Autodesk Inventor part; units mm, degrees
ref_plane "YZ Plane" through (0, 0, 0) normal (1, 0, 0) x (0, 1, 0)
ref_plane "XZ Plane" through (0, 0, 0) normal (0, 1, 0) x (-1, 0, 0)
ref_plane "XY Plane" through (0, 0, 0) normal (0, 0, 1) x (1, 0, 0)
sketch "Sketch1" plane through (0, 0, 0) normal (0, 0, 1) x (1, 0, 0)
  line L0 (-230, 170) -> (230, 170)
  line L1 (230, 170) -> (230, -170)
  line L2 (230, -170) -> (-230, -170)
  line L3 (-230, -170) -> (-230, 170)
  line L4 (130, 170) -> (230, 170)
  line L5 (230, 170) -> (230, -170)
  line L6 (230, -170) -> (130, -170)
  line L7 (130, -170) -> (130, 170)
  line L8 (-230, 170) -> (-130, 170)
  line L9 (-130, 170) -> (-130, -170)
  line L10 (-130, -170) -> (-230, -170)
  line L11 (-230, -170) -> (-230, 170)
  line L12 (-230, 170) -> (230, 170)
  line L13 (230, 170) -> (230, 95)
  line L14 (230, 95) -> (-230, 95)
  line L15 (-230, 95) -> (-230, 170)
  line L16 (-230, -95) -> (230, -95)
  line L17 (230, -95) -> (230, -170)
  line L18 (230, -170) -> (-230, -170)
  line L19 (-230, -170) -> (-230, -95)
  point P0 (0, 0)
  dimension "d0" = 460
  dimension "d1" = 340
  dimension "d2" = 170
  dimension "d3" = 230
  dimension "d4" = 100
  dimension "d5" = 100
  dimension "d6" = 75
  dimension "d7" = 75
extrude "Extrusion1" add sketch "Sketch1" along normal blind 25 contours L0 L9 L14 L3 | L0 L7 L14 L9 | L14 L9 L16 L3 | L0 L1 L14 L7 | L16 L9 L2 L3 | L14 L1 L16 L7 | L16 L7 L2 L9 | L16 L1 L2 L7
sketch "Sketch2" plane through (0, 0, 25) normal (0, 0, 1) x (1, 0, 0)
  line L0 (-92.0312, -155) -> (102.9688, -155)
  line L1 (102.9688, -155) -> (102.9688, -125)
  line L2 (102.9688, -125) -> (-92.0313, -125)
  line L3 (-92.0313, -125) -> (-92.0312, -155)
  line L4 (-230, -170) -> (230, -170)
  point P0 (0, 0)
  dimension "d10" = 30
  dimension "d11" = 195
  dimension "d12" = 15
extrude "Extrusion2" cut sketch "Sketch2" against normal blind 16
sketch "Sketch3" plane through (0, 0, 9) normal (0, 0, 1) x (1, 0, 0)
  line L0 (102.9688, -155) -> (-92.0312, -155)
  point P0 (0, 0)
  point P1 (-40, -140)
  point P2 (40, -140)
  dimension "d15" = 15
  dimension "d16" = 80
  dimension "d17" = 40
hole "Hole1" at (-40, -140, 9) at (40, -140, 9) direction (0, 0, -1) diameter 5.5 end through all
mirror "Mirror2" about plane through (0, 0, 0) normal (0, 1, 0) of "Extrusion2", "Hole1"
sketch "Sketch4" plane through (0, 0, 25) normal (0, 0, 1) x (1, 0, 0)
  line L0 (230, -170) -> (230, 170)
  line L1 (230, 170) -> (-230, 170)
  point P0 (0, 0)
  point P1 (180, 155)
  point P2 (215, 0)
  dimension "d25" = 15
  dimension "d26" = 15
  dimension "d27" = 50
hole "Hole2" at (180, 155, 25) at (215, 0, 25) direction (0, 0, -1) diameter 6.6 end through all counterbore diameter 18 counterbore depth 6.6
mirror "Mirror3" about plane through (0, 0, 0) normal (0, 1, 0) of "Hole2"
mirror "Mirror4" about plane through (0, 0, 0) normal (1, 0, 0) of "Hole2", "Mirror3"
properties part number "modified_xyStageMount"
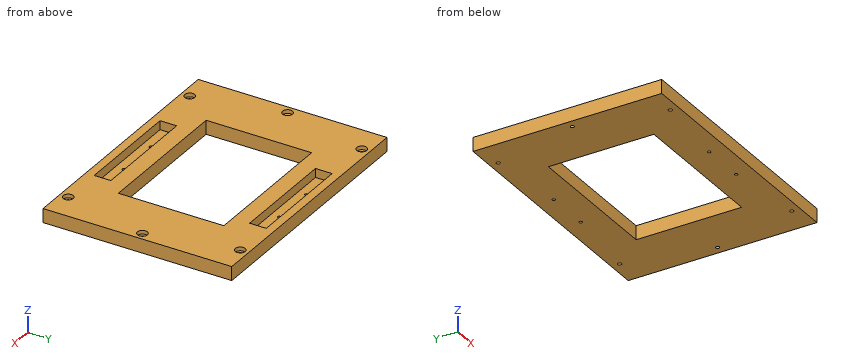
Build history of the part. All positions in model axes, mm. Coordinates: 2 decimals unless noted, no trailing zeros. Order: outer loops, then holes, each group sorted by start corner. A loop starts at its lowest first (then second) coordinate and runs counter-clockwise, first axis right, second up. Notation, with made-up numbers: (45.5, 75) - (52.5, 75) arc R12 cw to (52.5, 86) - close; hole circle Ø8 at (0.25, -4.75). An arc over 180 degrees is marked (long way). Put each result on its own line as item: value.
1. Saw through at A-A (z = 13.75). Give the number of separate pieces and of enclosed holes in the cut face, and give its area (3 significant figures).
Answer sheet:
separate pieces: 1
enclosed holes: 9
area: 95,100 mm^2
2. Saw through at B-B (y = 79). Write the cut outline in (x, z), and give its area (3 significant figures).
Answer sheet:
outline: (-230, 0) - (-130, 0) - (-130, 25) - (-230, 25) - close; (130, 0) - (230, 0) - (230, 25) - (130, 25) - close
area: 5,000 mm^2
3. Probe line 1 along X through (y, z) = (140, 5); line 2 along X through (y, z) = (0, 21); line 3 along Y through (x, z) = (-180, 10). List the from-to ranges inside material, lowest first. Write a range as [from, to].
Answer sheet:
line 1: x = [-230, -42.75], [-37.25, 37.25], [42.75, 230]
line 2: x = [-230, -224], [-206, -130], [130, 206], [224, 230]
line 3: y = [-170, -158.3], [-151.7, 151.7], [158.3, 170]
4. Saw through at C-C (x = 6). Write the cut outline in (y, z), and give its area (3 significant figures).
Answer sheet:
outline: (-170, 0) - (-95, 0) - (-95, 25) - (-125, 25) - (-125, 9) - (-155, 9) - (-155, 25) - (-170, 25) - close; (95, 0) - (170, 0) - (170, 25) - (155, 25) - (155, 9) - (125, 9) - (125, 25) - (95, 25) - close
area: 2,790 mm^2
5. Drop flat-ended pins along their axis: P1, Ø11, axis at x = 215, y = 0, coming from the +Z side; P2, Ø4, axis at x = -180, y = 155, coming from the +Z side. Give the stop position or say it passes through.
Answer sheet:
P1: stops at z = 18.4
P2: passes through
